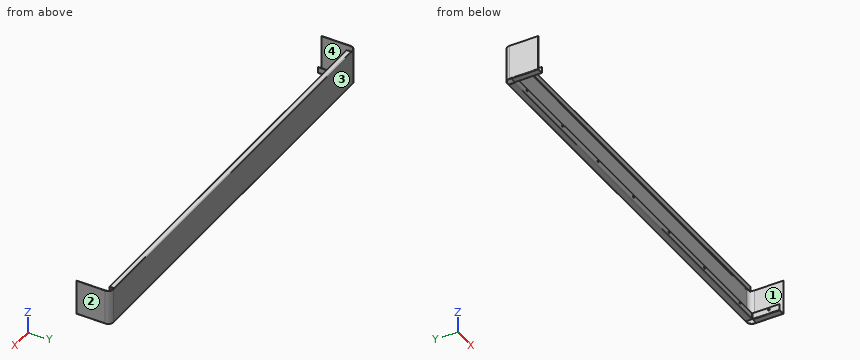
from build123d import *

# Parameters (mm, degrees)
BASE_FLANGE1_DEPTH             = 104
EDGE_FLANGE1_STRIP_W           = 6
EDGE_FLANGE1_STRIP_H           = 1
EDGE_FLANGE1_STRIP_CUT_DEPTH   = 1202
EDGE_FLANGE1_RELIEF_W          = 6.5
EDGE_FLANGE1_RELIEF_H          = 0.5
EDGE_FLANGE1_RELIEF_CUT_DEPTH  = 1
EDGE_FLANGE1_DEPTH             = 1202
EDGE_FLANGE2_STRIP_W           = 6
EDGE_FLANGE2_STRIP_H           = 1
EDGE_FLANGE2_STRIP_CUT_DEPTH   = 1202
EDGE_FLANGE2_DEPTH             = 1202
EDGE_FLANGE3_STRIP_W           = 6
EDGE_FLANGE3_STRIP_H           = 1
EDGE_FLANGE3_STRIP_CUT_DEPTH   = 80
EDGE_FLANGE3_RELIEF_W          = 6.5
EDGE_FLANGE3_RELIEF_H          = 0.5
EDGE_FLANGE3_RELIEF_CUT_DEPTH  = 1
EDGE_FLANGE3_DEPTH             = 80
EDGE_FLANGE4_STRIP_W           = 6
EDGE_FLANGE4_STRIP_H           = 1
EDGE_FLANGE4_STRIP_CUT_DEPTH   = 80
EDGE_FLANGE4_DEPTH             = 80
EDGE_FLANGE5_STRIP_W           = 6
EDGE_FLANGE5_STRIP_H           = 1
EDGE_FLANGE5_STRIP_CUT_DEPTH   = 1202
EDGE_FLANGE5_RELIEF_W          = 6.5
EDGE_FLANGE5_RELIEF_H          = 0.5
EDGE_FLANGE5_RELIEF_CUT_DEPTH  = 1
EDGE_FLANGE5_DEPTH             = 1202
SKETCH22_R                     = 3
CUT_EXTRUDE1_DEPTH             = 1
SKETCH23_R                     = 3
CUT_EXTRUDE2_DEPTH             = 3
CUT_EXTRUDE2_DIRECTION_2_REACH = 1234.474
EDGE_FLANGE6_STRIP_W           = 6
EDGE_FLANGE6_STRIP_H           = 1
EDGE_FLANGE6_STRIP_CUT_DEPTH   = 1202
EDGE_FLANGE6_DEPTH             = 1202


# Sheet-metal steps are written as plain solids
with BuildPart() as part:
    # Sketch1 → Base-Flange1 (new body)
    with BuildSketch(Plane.XY):
        with BuildLine():
            Line((-621, -100), (-621, -15))
            ThreePointArc((-621, -15), (-616.606601718, -4.393398282), (-606, 0))
            Line((-606, 0), (606, 0))
            ThreePointArc((606, 0), (616.606601718, -4.393398282), (621, -15))
            Line((621, -15), (621, -100))
            Line((621, -100), (622, -100))
            Line((622, -100), (622, -15))
            ThreePointArc((622, -15), (617.313708499, -3.686291501), (606, 1))
            Line((606, 1), (-606, 1))
            ThreePointArc((-606, 1), (-617.313708499, -3.686291501), (-622, -15))
            Line((-622, -15), (-622, -100))
            Line((-622, -100), (-621, -100))
        make_face()
    extrude(amount=BASE_FLANGE1_DEPTH)

    # Edge-Flange1 strip (across the edge) → Edge-Flange1 strip cut (cut)
    with BuildSketch(Plane(origin=(-601, 0, 0), x_dir=(0, 0, 1), z_dir=(1, 0, 0))):
        with Locations((-2, -0.5)):
            Rectangle(EDGE_FLANGE1_STRIP_W, EDGE_FLANGE1_STRIP_H)
    extrude(amount=EDGE_FLANGE1_STRIP_CUT_DEPTH, mode=Mode.SUBTRACT)

    # Edge-Flange1 relief (on the sheet) → Edge-Flange1 relief cut (cut)
    with BuildSketch(Plane(origin=(-601, 0, 1), x_dir=(0, 0, 1), z_dir=(0, -1, 0))):
        with Locations((-2.75, 0.25)):
            Rectangle(EDGE_FLANGE1_RELIEF_W, EDGE_FLANGE1_RELIEF_H)
        with Locations((-2.75, -1202.25)):
            Rectangle(EDGE_FLANGE1_RELIEF_W, EDGE_FLANGE1_RELIEF_H)
    extrude(amount=-EDGE_FLANGE1_RELIEF_CUT_DEPTH, mode=Mode.SUBTRACT)

    # Edge-Flange1 section (across the edge) → Edge-Flange1 (add)
    with BuildSketch(Plane(origin=(-601, 0, 0), x_dir=(0, 0, 1), z_dir=(1, 0, 0))):
        with BuildLine():
            Line((-1, 1), (-1, 19))
            Line((-1, 19), (0, 19))
            Line((0, 19), (0, 1))
            ThreePointArc((0, 1), (0.292893219, 0.292893219), (1, 0))
            Line((1, 0), (1, -1))
            ThreePointArc((1, -1), (-0.414213562, -0.414213562), (-1, 1))
        make_face()
    extrude(amount=EDGE_FLANGE1_DEPTH)

    # Edge-Flange2 strip (across the edge) → Edge-Flange2 strip cut (cut)
    with BuildSketch(Plane(origin=(-601, -19, 0), x_dir=(0, 1, 0), z_dir=(1, 0, 0))):
        with Locations((-1, -0.5)):
            Rectangle(EDGE_FLANGE2_STRIP_W, EDGE_FLANGE2_STRIP_H)
    extrude(amount=EDGE_FLANGE2_STRIP_CUT_DEPTH, mode=Mode.SUBTRACT)

    # Edge-Flange2 section (across the edge) → Edge-Flange2 (add)
    with BuildSketch(Plane(origin=(-601, -19, 0), x_dir=(0, 1, 0), z_dir=(1, 0, 0))):
        with BuildLine():
            Line((0, 1), (0, 18))
            Line((0, 18), (1, 18))
            Line((1, 18), (1, 1))
            ThreePointArc((1, 1), (1.292893219, 0.292893219), (2, 0))
            Line((2, 0), (2, -1))
            ThreePointArc((2, -1), (0.585786438, -0.414213562), (0, 1))
        make_face()
    extrude(amount=EDGE_FLANGE2_DEPTH)

    # Edge-Flange3 strip (across the edge) → Edge-Flange3 strip cut (cut)
    with BuildSketch(Plane(origin=(-621, -100, 0), x_dir=(0, 0, 1), z_dir=(0, 1, 0))):
        with Locations((-2, -0.5)):
            Rectangle(EDGE_FLANGE3_STRIP_W, EDGE_FLANGE3_STRIP_H)
    edge_flange3_strip_cut = extrude(amount=EDGE_FLANGE3_STRIP_CUT_DEPTH, mode=Mode.SUBTRACT)

    # Edge-Flange3 relief (on the sheet) → Edge-Flange3 relief cut (cut)
    with BuildSketch(Plane(origin=(-621, -100, 1), x_dir=(0, 0, 1), z_dir=(1, 0, 0))):
        with Locations((-2.75, -80.25)):
            Rectangle(EDGE_FLANGE3_RELIEF_W, EDGE_FLANGE3_RELIEF_H)
    edge_flange3_relief_cut = extrude(amount=-EDGE_FLANGE3_RELIEF_CUT_DEPTH, mode=Mode.SUBTRACT)

    # Edge-Flange3 section (across the edge) → Edge-Flange3 (add)
    with BuildSketch(Plane(origin=(-621, -100, 0), x_dir=(0, 0, 1), z_dir=(0, 1, 0))):
        with BuildLine():
            Line((-1, 1), (-1, 19))
            Line((-1, 19), (0, 19))
            Line((0, 19), (0, 1))
            ThreePointArc((0, 1), (0.292893219, 0.292893219), (1, 0))
            Line((1, 0), (1, -1))
            ThreePointArc((1, -1), (-0.414213562, -0.414213562), (-1, 1))
        make_face()
    edge_flange3 = extrude(amount=EDGE_FLANGE3_DEPTH)

    # Edge-Flange4 strip (across the edge) → Edge-Flange4 strip cut (cut)
    with BuildSketch(Plane(origin=(-602, -100, 0), x_dir=(-1, 0, 0), z_dir=(0, 1, 0))):
        with Locations((-1, -0.5)):
            Rectangle(EDGE_FLANGE4_STRIP_W, EDGE_FLANGE4_STRIP_H)
    edge_flange4_strip_cut = extrude(amount=EDGE_FLANGE4_STRIP_CUT_DEPTH, mode=Mode.SUBTRACT)

    # Edge-Flange4 section (across the edge) → Edge-Flange4 (add)
    with BuildSketch(Plane(origin=(-602, -100, 0), x_dir=(-1, 0, 0), z_dir=(0, 1, 0))):
        with BuildLine():
            Line((0, 1), (0, 18))
            Line((0, 18), (1, 18))
            Line((1, 18), (1, 1))
            ThreePointArc((1, 1), (1.292893219, 0.292893219), (2, 0))
            Line((2, 0), (2, -1))
            ThreePointArc((2, -1), (0.585786438, -0.414213562), (0, 1))
        make_face()
    edge_flange4 = extrude(amount=EDGE_FLANGE4_DEPTH)

    # Mirror1: Edge-Flange3 strip cut, Edge-Flange3 relief cut, Edge-Flange3, Edge-Flange4 strip cut, Edge-Flange4 across plane
    add(edge_flange3_strip_cut.mirror(Plane(origin=(0, 0, 0), x_dir=(0, 0, 1), z_dir=(1, 0, 0))), mode=Mode.SUBTRACT)
    add(edge_flange3_relief_cut.mirror(Plane(origin=(0, 0, 0), x_dir=(0, 0, 1), z_dir=(1, 0, 0))), mode=Mode.SUBTRACT)
    add(edge_flange3.mirror(Plane(origin=(0, 0, 0), x_dir=(0, 0, 1), z_dir=(1, 0, 0))))
    add(edge_flange4_strip_cut.mirror(Plane(origin=(0, 0, 0), x_dir=(0, 0, 1), z_dir=(1, 0, 0))), mode=Mode.SUBTRACT)
    add(edge_flange4.mirror(Plane(origin=(0, 0, 0), x_dir=(0, 0, 1), z_dir=(1, 0, 0))))

    # Edge-Flange5 strip (across the edge) → Edge-Flange5 strip cut (cut)
    with BuildSketch(Plane(origin=(601, 0, 104), x_dir=(0, 0, -1), z_dir=(-1, 0, 0))):
        with Locations((-1, -0.5)):
            Rectangle(EDGE_FLANGE5_STRIP_W, EDGE_FLANGE5_STRIP_H)
    extrude(amount=EDGE_FLANGE5_STRIP_CUT_DEPTH, mode=Mode.SUBTRACT)

    # Edge-Flange5 relief (on the sheet) → Edge-Flange5 relief cut (cut)
    with BuildSketch(Plane(origin=(601, 0, 102), x_dir=(0, 0, -1), z_dir=(0, -1, 0))):
        with Locations((-2.75, 0.25)):
            Rectangle(EDGE_FLANGE5_RELIEF_W, EDGE_FLANGE5_RELIEF_H)
        with Locations((-2.75, -1202.25)):
            Rectangle(EDGE_FLANGE5_RELIEF_W, EDGE_FLANGE5_RELIEF_H)
    extrude(amount=-EDGE_FLANGE5_RELIEF_CUT_DEPTH, mode=Mode.SUBTRACT)

    # Edge-Flange5 section (across the edge) → Edge-Flange5 (add)
    with BuildSketch(Plane(origin=(601, 0, 104), x_dir=(0, 0, -1), z_dir=(-1, 0, 0))):
        with BuildLine():
            Line((0, 1), (0, 15))
            Line((0, 15), (1, 15))
            Line((1, 15), (1, 1))
            ThreePointArc((1, 1), (1.292893219, 0.292893219), (2, 0))
            Line((2, 0), (2, -1))
            ThreePointArc((2, -1), (0.585786438, -0.414213562), (0, 1))
        make_face()
    extrude(amount=EDGE_FLANGE5_DEPTH)

    # Sketch22 → Cut-Extrude1 (cut)
    with BuildSketch(Plane.XZ.offset(19)):
        with Locations(Location((-540, 12, 0), (0, 0, 270))):
            Circle(SKETCH22_R)
        with Locations(Location((-360, 12, 0), (0, 0, 270))):
            Circle(SKETCH22_R)
        with Locations(Location((-180, 12, 0), (0, 0, 270))):
            Circle(SKETCH22_R)
        with Locations(Location((0, 12, 0), (0, 0, 270))):
            Circle(SKETCH22_R)
        with Locations(Location((180, 12, 0), (0, 0, 270))):
            Circle(SKETCH22_R)
        with Locations(Location((360, 12, 0), (0, 0, 270))):
            Circle(SKETCH22_R)
        with Locations(Location((540, 12, 0), (0, 0, 270))):
            Circle(SKETCH22_R)
    extrude(amount=-CUT_EXTRUDE1_DEPTH, mode=Mode.SUBTRACT)

    # Sketch23 → Cut-Extrude2 (cut)
    with BuildSketch(Plane.ZY.offset(-602)):
        with Locations(Location((12, -68, 0), (0, 0, 180))):
            Circle(SKETCH23_R)
    extrude(amount=-CUT_EXTRUDE2_DEPTH, mode=Mode.SUBTRACT)

    # Cut-Extrude2 direction 2: up to this face of the body (flat: up to its plane)
    cut_extrude2_direction_2_end = Plane(part.part.faces().sort_by_distance((-603, -60, 9.5))[0])
    # Sketch23 → Cut-Extrude2 direction 2 (cut, up to the picked face)
    with BuildSketch(Plane.ZY.offset(-602), mode=Mode.PRIVATE) as cut_extrude2_direction_2_sk1:
        with Locations(Location((12, -68, 0), (0, 0, 180))):
            Circle(SKETCH23_R)
    cut_extrude2_direction_2_tool1 = split(extrude(cut_extrude2_direction_2_sk1.sketch, amount=CUT_EXTRUDE2_DIRECTION_2_REACH, mode=Mode.PRIVATE), bisect_by=cut_extrude2_direction_2_end, keep=Keep.BOTH, mode=Mode.PRIVATE)
    add(cut_extrude2_direction_2_tool1.solids().sort_by(Axis((602, -68, 12), (-1, 0, 0)))[0], mode=Mode.SUBTRACT)

    # Edge-Flange6 strip (across the edge) → Edge-Flange6 strip cut (cut)
    with BuildSketch(Plane(origin=(601, -15, 103), x_dir=(0, 1, 0), z_dir=(-1, 0, 0))):
        with Locations((-1, -0.5)):
            Rectangle(EDGE_FLANGE6_STRIP_W, EDGE_FLANGE6_STRIP_H)
    extrude(amount=EDGE_FLANGE6_STRIP_CUT_DEPTH, mode=Mode.SUBTRACT)

    # Edge-Flange6 section (across the edge) → Edge-Flange6 (add)
    with BuildSketch(Plane(origin=(601, -15, 103), x_dir=(0, 1, 0), z_dir=(-1, 0, 0))):
        with BuildLine():
            Line((0, 1), (0, 17))
            Line((0, 17), (1, 17))
            Line((1, 17), (1, 1))
            ThreePointArc((1, 1), (1.292893219, 0.292893219), (2, 0))
            Line((2, 0), (2, -1))
            ThreePointArc((2, -1), (0.585786438, -0.414213562), (0, 1))
        make_face()
    extrude(amount=EDGE_FLANGE6_DEPTH)


solid = part.part
Could you check a few things on this model? Use its own coordinates, in mm. Face numbers are marked on the shaded views. Give positions to 0.01 mm unless a question says otherwise; leave off trailing zeros. Order: outer loops, then holes, each group sorted by start corner. A loop starts at its lowest first (then second) coordinate and runs counter-clockwise, first axis right, second up. Notation, with made-up numbers: (-10, 58) - (7, 58) arc R22 ccw to (7, 81) - close; hole circle Ø11 at (26.25, 19.25). An arc over 180 degrees is marked (long way). One line per item, written item: value. Start each with the question number.
1. For P1, Ø0.6, axis at x = 601, y = 0.5, coming from the -Z side; P2, Ø0.8, axis at x = -602.5, y = -47.5, coming from the +Z side; P3, Ø6, axis at x = -155, z = 67.5, coming from the -Y side; P4, Ø10, axis at x = 608, y = -10, coming from the -Z side, each with a flat end and sliding along its axis, tell me the tip position at first contact or that it passes through.
2. Imagine slicing it at B-B on z = 64.5. List the corners of the cut face in (x, y) for me, plus the area to 3 significant figures.
3. Imagine slicing it at C-C on x = -270.5. List the corners of the cut face in (y, z) for me, plus the area to 3 significant figures.
4. Thinking about a two-plate mould opening in X: for the marked faces 1, 2, 3 and 4, which applies, +X half, -X half, draft (parallel to the pull), parting line (faces both ways), or undercut?
5. If I drill on probe 1 along X at (y, z) = (-50, 9); probe 2 along X at (y, z) = (-91.5, 99.5); probe 3 along Y at (x, z) = (-510.5, 8), over which ranges is the centre line in solid material (lowest first)?
6. Imagine slicing it at A-A on y = -88. List the corners of the cut face in (x, z) for me, plus the area to 3 significant figures.
Values:
1. P1: z = -0.6
1. P2: z = 18
1. P3: y = 0
1. P4: through
2. outline: (-622, -100) - (-621, -100) - (-621, -15) arc R15 cw to (-606, 0) - (606, 0) arc R15 cw to (621, -15) - (621, -100) - (622, -100) - (622, -15) arc R16 ccw to (606, 1) - (-606, 1) arc R16 ccw to (-622, -15) - close
2. area: 1,430 mm²
3. outline: (-19, 1) arc R2 ccw to (-17, -1) - (-1, -1) arc R2 ccw to (1, 1) - (1, 102) arc R2 ccw to (-1, 104) - (-13, 104) arc R2 ccw to (-15, 102) - (-15, 86) - (-14, 86) - (-14, 102) arc R1 cw to (-13, 103) - (-1, 103) arc R1 cw to (0, 102) - (0, 1) arc R1 cw to (-1, 0) - (-17, 0) arc R1 cw to (-18, 1) - (-18, 18) - (-19, 18) - close
3. area: 171 mm²
4. face 1: undercut
4. face 2: +X half
4. face 3: draft
4. face 4: undercut
5. probe 1: -622 to -621, -603 to -602, 602 to 603, 621 to 622
5. probe 2: -622 to -621, 621 to 622
5. probe 3: -19 to -18, 0 to 1
6. outline: (-622, 1) arc R2 ccw to (-620, -1) - (-604, -1) arc R2 ccw to (-602, 1) - (-602, 18) - (-603, 18) - (-603, 1) arc R1 cw to (-604, 0) - (-620, 0) arc R1 cw to (-621, 1) - (-621, 104) - (-622, 104) - close; (602, 1) arc R2 ccw to (604, -1) - (620, -1) arc R2 ccw to (622, 1) - (622, 104) - (621, 104) - (621, 1) arc R1 cw to (620, 0) - (604, 0) arc R1 cw to (603, 1) - (603, 18) - (602, 18) - close
6. area: 281 mm²
